Input: part model. Units: mm. Frame: model coordinates. A direction names the side the tool comes from. Give positions to 0.01 mm unless a question says otherwise; leave off trailing zeros. Order: outer loops, then holes, each group sorted by start corner. A loop starts at its lowest first (then second) coordinate and runs counter-clockwise, first axis right, second up. Notation, with made-up numbers: (50, 87) -> (77, 87) arc R24 ccw to (77, 118) -> close; hole circle Ø7 at (-1, -30.5). An arc over 180 degrees is marked (long way). Use a Markdown table: item, result. Add a question column.
from build123d import *

# Parameters (mm, degrees)
F0_W     = 3
F0_H     = 4.5
F0_W_2   = 6
F1_DEPTH = 4
F2_DEPTH = 1.5
F3_DEPTH = 4
F4_DEPTH = 15.5
F5_R     = 3


with BuildPart() as f1:
    # F0 (on Top) → F1 (new body)
    with BuildSketch(Plane.XY):
        Polygon((12, -7.5), (12, 7.5), (9, 7.5), (3, 7.5), (-3, 7.5), (-9, 7.5), (-12, 7.5), (-12, -7.5), (-9, -7.5), (-3, -7.5), (3, -7.5), (9, -7.5), align=None)
        with BuildLine():
            ThreePointArc((7, -3), (6.1213203436, -5.1213203436), (4, -6))
            Line((4, -6), (-4, -6))
            ThreePointArc((-4, -6), (-6.1213203436, -5.1213203436), (-7, -3))
            Line((-7, -3), (-7, 3))
            ThreePointArc((-7, 3), (-6.1213203436, 5.1213203436), (-4, 6))
            Line((-4, 6), (4, 6))
            ThreePointArc((4, 6), (6.1213203436, 5.1213203436), (7, 3))
            Line((7, 3), (7, -3))
        make_face(mode=Mode.SUBTRACT)
        with Locations((10.5, -9.75)):
            Rectangle(F0_W, F0_H)
        with Locations((6, -9.75)):
            Rectangle(F0_W_2, F0_H)
        with Locations((0, -9.75)):
            Rectangle(F0_W_2, F0_H)
        with Locations((-6, -9.75)):
            Rectangle(F0_W_2, F0_H)
        with Locations((-10.5, -9.75)):
            Rectangle(F0_W, F0_H)
        with Locations((-10.5, 9.75)):
            Rectangle(F0_W, F0_H)
        with Locations((-6, 9.75)):
            Rectangle(F0_W_2, F0_H)
        with Locations((0, 9.75)):
            Rectangle(F0_W_2, F0_H)
        with Locations((6, 9.75)):
            Rectangle(F0_W_2, F0_H)
        with Locations((10.5, 9.75)):
            Rectangle(F0_W, F0_H)
    extrude(amount=-F1_DEPTH)

    # F0 (on Top) → F2 (join)
    with BuildSketch(Plane.XY):
        Polygon((12, -7.5), (12, 7.5), (9, 7.5), (3, 7.5), (-3, 7.5), (-9, 7.5), (-12, 7.5), (-12, -7.5), (-9, -7.5), (-3, -7.5), (3, -7.5), (9, -7.5), align=None)
        with BuildLine():
            ThreePointArc((7, -3), (6.1213203436, -5.1213203436), (4, -6))
            Line((4, -6), (-4, -6))
            ThreePointArc((-4, -6), (-6.1213203436, -5.1213203436), (-7, -3))
            Line((-7, -3), (-7, 3))
            ThreePointArc((-7, 3), (-6.1213203436, 5.1213203436), (-4, 6))
            Line((-4, 6), (4, 6))
            ThreePointArc((4, 6), (6.1213203436, 5.1213203436), (7, 3))
            Line((7, 3), (7, -3))
        make_face(mode=Mode.SUBTRACT)
        with BuildLine():
            Line((-4, -6), (4, -6))
            ThreePointArc((4, -6), (6.1213203436, -5.1213203436), (7, -3))
            Line((7, -3), (7, 3))
            ThreePointArc((7, 3), (6.1213203436, 5.1213203436), (4, 6))
            Line((4, 6), (-4, 6))
            ThreePointArc((-4, 6), (-6.1213203436, 5.1213203436), (-7, 3))
            Line((-7, 3), (-7, -3))
            ThreePointArc((-7, -3), (-6.1213203436, -5.1213203436), (-4, -6))
        make_face()
    extrude(amount=F2_DEPTH)

    # F0 (on Top) → F3 (join)
    with BuildSketch(Plane.XY):
        with Locations((10.5, 9.75)):
            Rectangle(F0_W, F0_H)
        with Locations((0, 9.75)):
            Rectangle(F0_W_2, F0_H)
        with Locations((-10.5, 9.75)):
            Rectangle(F0_W, F0_H)
        with Locations((-10.5, -9.75)):
            Rectangle(F0_W, F0_H)
        with Locations((0, -9.75)):
            Rectangle(F0_W_2, F0_H)
        with Locations((10.5, -9.75)):
            Rectangle(F0_W, F0_H)
    extrude(amount=F3_DEPTH)

    # F0 (on Top) → F4 (join)
    with BuildSketch(Plane.XY):
        with Locations((-6, 9.75)):
            Rectangle(F0_W_2, F0_H)
        with Locations((6, 9.75)):
            Rectangle(F0_W_2, F0_H)
        with Locations((6, -9.75)):
            Rectangle(F0_W_2, F0_H)
        with Locations((-6, -9.75)):
            Rectangle(F0_W_2, F0_H)
    extrude(amount=F4_DEPTH)

    # F5
    f5_edges = [f1.edges().sort_by_distance(p)[0] for p in [
        (6, 12, 15.5),
        (-6, 12, 15.5),
        (6, -12, 15.5),
        (-6, -12, 15.5),
    ]]
    fillet(f5_edges, radius=F5_R)


solid = f1.part
Q1. Section query A-A (z = 7.25). Return loops of the section in (x, y), plus the area to 3 significant figures.
Q2. Section query D-D (y = 8.25). Return loops of the section in (x, z), plus the area to 3 significant figures.
Q3. First-contact query: pin 1 (2 mm diameter, centred on y = -10.5, z = 11, fed in from +X); pin 2 (10 mm diameter, centred on x = 7.5, z = 13.5, fed in from -Y); pin 3 (5 mm diameter, centred on y = 10.5, z = 8, fed in from -X); pin 4 (3.5 mm diameter, centred on x = -10.5, y = 10.5, fed in from +Z). Flat tips, straight axial feed; report the tip coordinate or a pass-through.
Q4. Ray query, line 1 (Y direction, x = -8.5, z = 12.5); line 2 (X direction, y = 10.25, z = 6.75); line 3 (Z direction, x = -11, y = -8.75). Return the intervals inside material, ascending.
Q5. Access query for faces 1 (the cylindrical face through (6.1, 5.14, -1.97)), 2 (the flat face through (-6, 8, 15.5)), 3 (the flat face through (-0.2, -7.5, 3.7)), 4 (the flat face through (3, 10, 10)). Directions: +Z, -Z, +X, -X, +Y, -Y. A direction counts if a zero-diameter tool reaches every point of the face in a straight line with its end or side. Return the directions, or none.
Q6. Section query C-C (y = 1.5). Return loops of the section in (x, z).
Q7. Section query B-B (x = -2.5). Return loops of the section in (y, z), plus the area to 4 significant figures.
Q8. Draft query along X for faces 5 (the flat face through (6, 8, 15.5)), 6 (the flat face through (-12, 0, -1)), 7 (the flat face through (7, 0, -2)). Return one class per face: +X half, -X half, draft (parallel to the pull), parting line (faces both ways), or undercut.
Solution:
| question | item | result |
|---|---|---|
| 1 | outline | (-9, -12) -> (-3, -12) -> (-3, -7.5) -> (-9, -7.5) -> close; (-9, 7.5) -> (-3, 7.5) -> (-3, 12) -> (-9, 12) -> close; (3, -12) -> (9, -12) -> (9, -7.5) -> (3, -7.5) -> close; (3, 7.5) -> (9, 7.5) -> (9, 12) -> (3, 12) -> close |
| 1 | area | 108 mm² |
| 2 | outline | (-12, -4) -> (12, -4) -> (12, 4) -> (9, 4) -> (9, 15.5) -> (3, 15.5) -> (3, 4) -> (-3, 4) -> (-3, 15.5) -> (-9, 15.5) -> (-9, 4) -> (-12, 4) -> close |
| 2 | area | 330 mm² |
| 3 | pin 1 | stops at x = 9 |
| 3 | pin 2 | stops at y = -12 |
| 3 | pin 3 | stops at x = -9 |
| 3 | pin 4 | stops at z = 15.44 |
| 4 | line 1 | y = -12 to -7.5, 7.5 to 12 |
| 4 | line 2 | x = -9 to -3, 3 to 9 |
| 4 | line 3 | z = -4 to 4 |
| 5 | face 1 | -Z |
| 5 | face 2 | +Z, +X, -X, +Y, -Y |
| 5 | face 3 | +Z, +X, -X |
| 5 | face 4 | +Z, +Y, -Y |
| 6 | outline | (-12, -4) -> (-7, -4) -> (-7, 0) -> (7, 0) -> (7, -4) -> (12, -4) -> (12, 1.5) -> (-12, 1.5) -> close |
| 7 | outline | (-12, -4) -> (-6, -4) -> (-6, 0) -> (6, 0) -> (6, -4) -> (12, -4) -> (12, 4) -> (7.5, 4) -> (7.5, 1.5) -> (-7.5, 1.5) -> (-7.5, 4) -> (-12, 4) -> close |
| 7 | area | 106.5 mm² |
| 8 | face 5 | draft |
| 8 | face 6 | -X half |
| 8 | face 7 | undercut |
